Design review of the part built by this model. Coordinates are the model's own, in mm. Face numbers are marked on the shaded views. A direction names the side the tool comes from. Coordinates: 2 decimals unless noted, no trailing zeros. Write each loop counter-clockwise with the first axis right and the second up, starting at its lowest first coordinate (ties: lowest second). Pieces come first, ordered by that corner, then holes.
Q1. Add section A-A, the plane x = -52. Give the boundary of the cut face in (y, z).
Q2. Clearance check with flat-ended pins moving along their axes: pin 1 Ø2 at (x, y) = (97, -11.5) entering from +Z; pin 2 Ø1.5 at (y, z) = (-39.5, -51.5) entering from +X; pin 3 Ø12.5 at (x, y) = (51.5, -17) entering from +Z; pin 4 Ø4 at (y, z) = (-53.5, -53) entering from +X. State where each tip first meets the part, or that it passes through.
Q3. Add section C-C, the plane z = -5. Give the boundary of the cut face in (x, y), plus the area to 3 significant figures.
Q4. Add section D-D, the plane y = -19. Give the number of separate pieces and of enclosed holes in the cut face, plus the area to 3 significant figures.
Q5. The part is to be moulded in two halves that separate along Z. For the marked faces 3, 4, 5 and 6, say which applies: +Z half, -Z half, draft (parallel to the pull), parting line (faces both ways), or undercut.
Q6. Add section B-B, the plane x = -97.5. Give the boundary of the cut face in (y, z).
Q7. To check wall thickness, follow probe 1 along X at (y, z) = (-33, -51.5); probe 2 along Z at (x, y) = (57.5, -12); probe 3 along Z at (x, y) = (-52, -17). State the ranges of each line that lie inside material, in increasing order.
Q8. Machinability: for the marked faces 1 and 2, which of the approach directions +Z, -Z, +X, -X, +Y, -Y give a long, thin tool a straight path to every point of the face, cutting with its end or side? Answer none if there is none.
from build123d import *

# Parameters (mm, degrees)
F1_DEPTH      = 70
F1_DEPTH_BACK = 70
F2_R          = 7
F3_DEPTH      = 4
F4_W          = 135
F4_H          = 50
F5_DEPTH      = 3
F7_DEPTH      = 8
F8_R          = 20
F9_DEPTH      = 4
F10_W         = 60
F10_H         = 4
F11_DEPTH     = 25
F12_W         = 54
F12_H         = 19
F13_DEPTH     = 2
F14_R         = 5


with BuildPart() as f1:
    # F0 (on Right) → F1 (new body, two sides)
    with BuildSketch(Plane.YZ) as f1_sk:
        with BuildLine():
            Line((0, -55), (0, 51))
            ThreePointArc((0, 51), (-0.8786796564, 53.1213203436), (-3, 54))
            Line((-3, 54), (-35, 54))
            Line((-35, 54), (-35, 50))
            Line((-35, 50), (-8, 50))
            ThreePointArc((-8, 50), (-5.8786796564, 49.1213203436), (-5, 47))
            Line((-5, 47), (-5, -50))
            Line((-5, -50), (-60, -50))
            Line((-60, -50), (-60, -58))
            Line((-60, -58), (-3, -58))
            ThreePointArc((-3, -58), (-0.8786796564, -57.1213203436), (0, -55))
        make_face()
    extrude(amount=-F1_DEPTH)
    extrude(f1_sk.sketch, amount=F1_DEPTH_BACK)

    # F2 (on face) → F3 (cut, through all)
    with BuildSketch(Plane.XY.offset(54)):
        with BuildLine():
            Line((55, -11), (20, -11))
            ThreePointArc((20, -11), (12, -19), (20, -27))
            Line((20, -27), (55, -27))
            ThreePointArc((55, -27), (63, -19), (55, -11))
        make_face()
        with Locations((-16, -19)):
            Circle(F2_R)
        with Locations((-52, -19)):
            Circle(F2_R)
    extrude(amount=-F3_DEPTH, mode=Mode.SUBTRACT)

    # F4 (on face) → F5 (cut)
    with BuildSketch(Plane.XY.offset(-50)):
        with Locations((0, -32.5)):
            Rectangle(F4_W, F4_H)
    extrude(amount=-F5_DEPTH, mode=Mode.SUBTRACT)

    # F6 (on face) → F7 (join)
    with BuildSketch(Plane.XY.offset(-50)):
        with BuildLine():
            Line((70, -32), (70, -49))
            Line((70, -49), (75.8840336788, -49))
            ThreePointArc((75.8840336788, -49), (71.5126081163, -40.9947464157), (70, -32))
        make_face()
        with BuildLine():
            ThreePointArc((70, -32), (71.5126081163, -40.9947464157), (75.8840336788, -49))
            ThreePointArc((75.8840336788, -49), (106.4947464157, -57.9873918837), (125, -32))
            ThreePointArc((125, -32), (106.4947464157, -6.0126081163), (75.8840336788, -15))
            ThreePointArc((75.8840336788, -15), (71.5126081163, -23.0052535843), (70, -32))
        make_face()
        with BuildLine():
            Line((70, -15), (70, -32))
            ThreePointArc((70, -32), (71.5126081163, -23.0052535843), (75.8840336788, -15))
            Line((75.8840336788, -15), (70, -15))
        make_face()
        with BuildLine():
            ThreePointArc((-75.8840336788, -49), (-71.5126081163, -40.9947464157), (-70, -32))
            ThreePointArc((-70, -32), (-71.5126081163, -23.0052535843), (-75.8840336788, -15))
            ThreePointArc((-75.8840336788, -15), (-125, -32), (-75.8840336788, -49))
        make_face()
        with BuildLine():
            Line((-70, -49), (-70, -32))
            ThreePointArc((-70, -32), (-71.5126081163, -40.9947464157), (-75.8840336788, -49))
            Line((-75.8840336788, -49), (-70, -49))
        make_face()
        with BuildLine():
            ThreePointArc((-75.8840336788, -15), (-71.5126081163, -23.0052535843), (-70, -32))
            Line((-70, -32), (-70, -15))
            Line((-70, -15), (-75.8840336788, -15))
        make_face()
    extrude(amount=-F7_DEPTH)

    # F8 (on face) → F9 (cut)
    with BuildSketch(Plane.XY.offset(-50)):
        with Locations((-97.5, -32)):
            Circle(F8_R)
        with Locations((97.5, -32)):
            Circle(F8_R)
    extrude(amount=-F9_DEPTH, mode=Mode.SUBTRACT)

    # F10 (on face) → F11 (join)
    with BuildSketch(Plane.XZ.offset(5)):
        with Locations((40, 2)):
            Rectangle(F10_W, F10_H)
    extrude(amount=F11_DEPTH)

    # F12 (on face) → F13 (cut)
    with BuildSketch(Plane.XY.offset(4)):
        with Locations((40, -17.5)):
            Rectangle(F12_W, F12_H)
    extrude(amount=-F13_DEPTH, mode=Mode.SUBTRACT)

    # F14
    f14_edges = [f1.edges().sort_by_distance(p)[0] for p in [
        (-70, -35, 52),
        (70, -35, 52),
    ]]
    fillet(f14_edges, radius=F14_R)


solid = f1.part
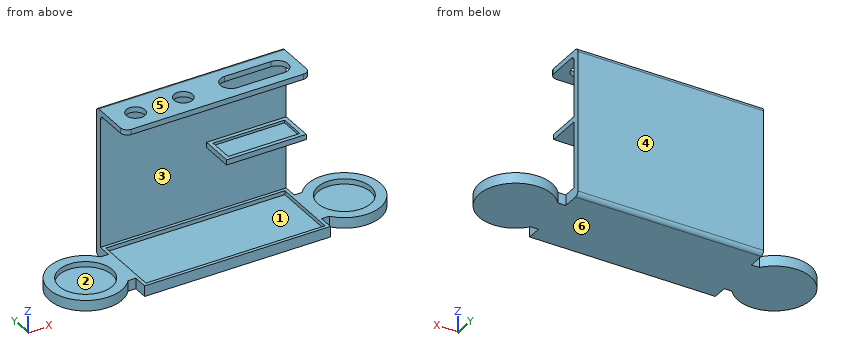
Here are the results:
1. outline: (-60, -58) - (-3, -58) arc R3 ccw to (0, -55) - (0, 51) arc R3 ccw to (-3, 54) - (-12, 54) - (-12, 50) - (-8, 50) arc R3 cw to (-5, 47) - (-5, -50) - (-7.5, -50) - (-7.5, -53) - (-57.5, -53) - (-57.5, -50) - (-60, -50) - close; (-35, 50) - (-26, 50) - (-26, 54) - (-35, 54) - close
2. pin 1: stops at z = -50
2. pin 2: stops at x = 124.16
2. pin 3: stops at z = 54
2. pin 4: stops at x = 116.89
3. outline: (-70, -5) - (70, -5) - (70, 0) - (-70, 0) - close
3. area: 700 mm2
4. separate pieces: 6
4. enclosed holes: 0
4. area: 1,680 mm2
5. face 3: undercut
5. face 4: draft
5. face 5: +Z half
5. face 6: -Z half
6. outline: (-59.5, -58) - (-4.5, -58) - (-4.5, -50) - (-12, -50) - (-12, -54) - (-52, -54) - (-52, -50) - (-59.5, -50) - close
7. probe 1: x = -124.98 to -117.47, -77.53 to -67.5, 67.5 to 77.53, 117.47 to 124.98
7. probe 2: z = -58 to -53, 0 to 2
7. probe 3: z = -58 to -53
8. face 1: none
8. face 2: +Z
